For this review, use the dimensioned drawing (mm, ordinates from the lowest corner) and the shaded views. Round coordinates to 2 decimals unless told otherwise and drop trailing zeros. Order: outer loops, then holes, each group sorted by start corner. A loop starts at its lowest first (then second) coordinate and runs counter-clockwise, first axis right, second up. Notation, with made-up numbers: M 39.5,38 L 43.5,38 A31 ccw 43.5,76 Z; hole C -30,32 d1. An arc over 180 degrees is marked long. Put each result on its own line as item: value.
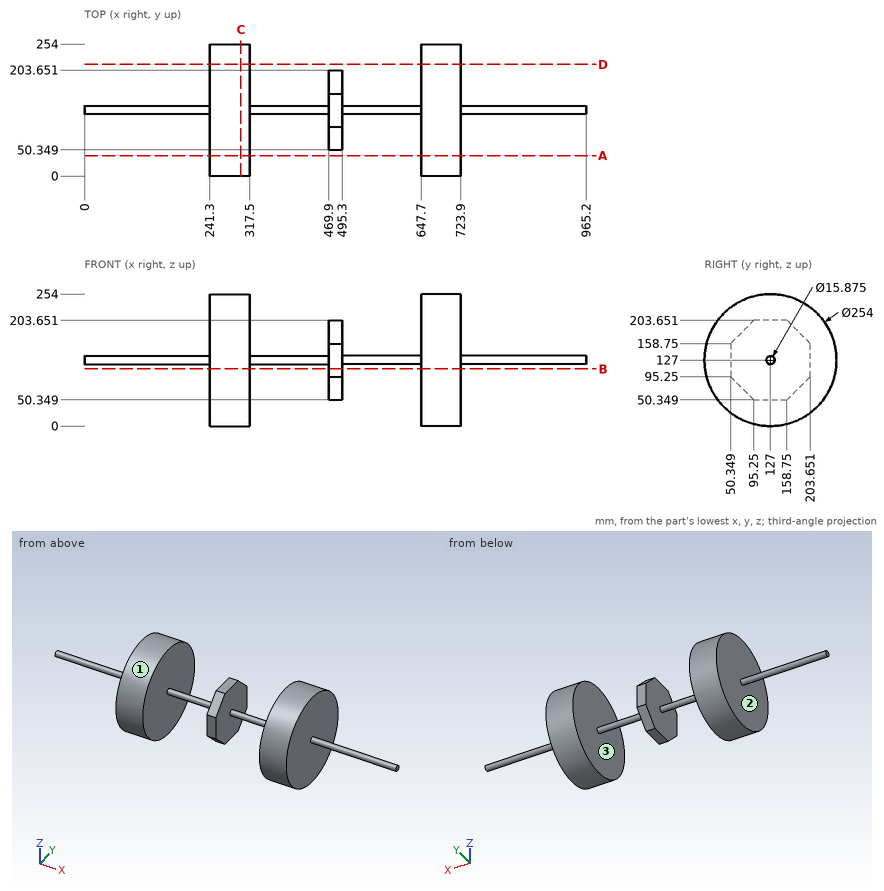
(1) Add section D-D on y = 215. Give the boundary of the cut face in (x, z).
A:
outline: M 241.3,35.43 L 317.5,35.43 L 317.5,218.57 L 241.3,218.57 Z; M 647.7,35.43 L 723.9,35.43 L 723.9,218.57 L 647.7,218.57 Z
(2) Add section A-A on y = 39.5. Give the boundary of the cut face in (x, z), then the cut area to 3 significant figures.
A:
outline: M 241.3,34.95 L 317.5,34.95 L 317.5,219.05 L 241.3,219.05 Z; M 647.7,34.95 L 723.9,34.95 L 723.9,219.05 L 647.7,219.05 Z
area: 28,100 mm2
(3) To check wall thickness, follow L1, parallel to X at y = 101.5, z = 168.5; L2, parallel to X at y = 212, z = 128; L3, parallel to Z at x = 461, y = 128. State the ranges of each line that lie inside material, in increasing order.
A:
L1: x = 241.3 to 317.5, 469.9 to 495.3, 647.7 to 723.9
L2: x = 241.3 to 317.5, 647.7 to 723.9
L3: z = 119.13 to 134.87
(4) Add section C-C on x = 300.5. Give the boundary of the cut face in (y, z).
A:
outline: C 127,127 d254
(5) Draft analysis for pull direction X (two halves, no side actions). For the marked faces 1, 2 and 3, state which applies: released by +X, released by -X, zero draft, split by the parting line, or undercut.
A:
face 1: zero draft
face 2: released by -X
face 3: undercut
(6) Insertion check: pin 1 Ø2 at (y, z) = (87.5, 168) entering from +X; pin 2 Ø4 at (x, y) = (217.5, 131.5) entering from -Z; pin 3 Ø12.5 at (x, y) = (486, 134) entering from -Z; pin 4 Ø1 at (x, y) = (113, 135.5) entering from +Z. Each pin has a flat end and moves straight along its axis. Give the tip position at first contact, or say it passes through.
A:
pin 1: stops at x = 723.9
pin 2: stops at z = 119.47
pin 3: stops at z = 50.35
pin 4: passes through
(7) Add section B-B on z = 110. Give the boundary of the cut face in (x, y).
A:
outline: M 241.3,1.14 L 317.5,1.14 L 317.5,252.86 L 241.3,252.86 Z; M 469.9,50.35 L 495.3,50.35 L 495.3,203.65 L 469.9,203.65 Z; M 647.7,1.14 L 723.9,1.14 L 723.9,252.86 L 647.7,252.86 Z
